from build123d import *

# Parameters (mm, degrees)
SKETCH_1_W      = 22.5
SKETCH_1_H      = 12.5
EXTRUDE_1_DEPTH = 17
SKETCH_2_W      = 32
SKETCH_2_H      = 12.5
SKETCH_2_R      = 1.5
EXTRUDE_2_DEPTH = 1.5
SKETCH_3_W      = 22.5
SKETCH_3_H      = 12.5
EXTRUDE_3_DEPTH = 4
SKETCH_4_R      = 5.5
EXTRUDE_4_DEPTH = 6.5
SKETCH_5_R      = 2.5
EXTRUDE_5_DEPTH = 3.5


with BuildPart() as part:
    # 草图1 → 凸台-拉伸1 (new body)
    with BuildSketch(Plane(origin=(0, 0, 0), x_dir=(1, 0, 0), z_dir=(0, 1, 0))):
        with Locations((11.25, -6.25)):
            Rectangle(SKETCH_1_W, SKETCH_1_H)
    extrude(amount=EXTRUDE_1_DEPTH)

    # 草图2 → 凸台-拉伸2 (add)
    with BuildSketch(Plane(origin=(0, 17, 0), x_dir=(1, 0, 0), z_dir=(0, 1, 0))):
        with Locations((11.25, -6.25)):
            Rectangle(SKETCH_2_W, SKETCH_2_H)
        with Locations(Location((-2.75, -6.25, 0), (0, 0, 270))):
            Circle(SKETCH_2_R, mode=Mode.SUBTRACT)
        with Locations(Location((25.25, -6.25, 0), (0, 0, 270))):
            Circle(SKETCH_2_R, mode=Mode.SUBTRACT)
    extrude(amount=EXTRUDE_2_DEPTH)

    # 草图3 → 凸台-拉伸3 (add)
    with BuildSketch(Plane(origin=(0, 18.5, 0), x_dir=(1, 0, 0), z_dir=(0, 1, 0))):
        with Locations((11.25, -6.25)):
            Rectangle(SKETCH_3_W, SKETCH_3_H)
    extrude(amount=EXTRUDE_3_DEPTH)

    # 草图4 → 凸台-拉伸4 (add)
    with BuildSketch(Plane(origin=(0, 22.5, 0), x_dir=(1, 0, 0), z_dir=(0, 1, 0))):
        with Locations(Location((17.25, -6.25, 0), (0, 0, 17.341442803))):
            Circle(SKETCH_4_R)
    extrude(amount=EXTRUDE_4_DEPTH)

    # 草图5 → 凸台-拉伸5 (add)
    with BuildSketch(Plane(origin=(0, 29, 0), x_dir=(1, 0, 0), z_dir=(0, 1, 0))):
        with Locations(Location((17.25, -6.25, 0), (0, 0, 270))):
            Circle(SKETCH_5_R)
    extrude(amount=EXTRUDE_5_DEPTH)


solid = part.part
Could you check a few things on this model? Use its own coordinates, in mm. A direction names the side the tool comes from. Round coordinates to 2 decimals unless told otherwise and drop trailing zeros. Loops run counter-clockwise (first coordinate to the right, second up) from the corner with the lowest first, then second, coordinate; pieces in that order, holes last. Notation, with made-up numbers: (-35, 18.5) - (-6, 18.5) arc R12 cw to (-6, 25.5) - close; hole circle Ø9 at (85.5, 39.25). An arc over 180 degrees is marked (long way). Write item = value, one per line.
1) I need wall thicknesses on line 1 along X through (y, z) = (17.9, 6.25); line 2 along Y through (x, z) = (-1.5, 2.75); line 3 along Y through (x, z) = (19.5, 11.5). Which ranges of each line are inside material? Lowest first, please. Write a range as from..to.
Computed:
line_1 = -4.75..-4.25, -1.25..23.75, 26.75..27.25
line_2 = 17..18.5
line_3 = 0..22.5
2) Imagine slicing it at B-B (x = -2.75). Please give me the cut outline in (y, z).
Computed:
outline = (17, 0) - (18.5, 0) - (18.5, 4.75) - (17, 4.75) - close; (17, 7.75) - (18.5, 7.75) - (18.5, 12.5) - (17, 12.5) - close
3) Imagine slicing it at C-C (y = 28.5). Please give me the cut outline in (x, z), and give its area (3 significant figures).
Computed:
outline = circle Ø11 at (17.25, 6.25)
area = 95.0 mm2
4) Imagine slicing it at D-D (x = 17.25). Please give me the cut outline in (y, z), and give its area (3 significant figures).
Computed:
outline = (0, 0) - (22.5, 0) - (22.5, 0.75) - (29, 0.75) - (29, 3.75) - (32.5, 3.75) - (32.5, 8.75) - (29, 8.75) - (29, 11.75) - (22.5, 11.75) - (22.5, 12.5) - (0, 12.5) - close
area = 370 mm2
5) On a 3-axis mill with a long thin cutter (end or side, diameter ignored), from which of +Z, -Z, +X, -X, +Y, -Y can I reach the whole of each face in a straight line? I mean faces 1 (the flat face through (0, 20, 6)), 2 (the flat face through (22.5, 20, 6)), 3 (the cylindrical face through (19.36, 30.73, 7.59)). Say none if no direction works.
Computed:
face_1 = +Z, -Z, -X, +Y
face_2 = +Z, -Z, +X
face_3 = +Y
6) If we mould it in two halves opening along Z, with no side actions, what happens to faces 4 (the flat face through (-1.9, 17, 4.8)), 5 (the flat face through (11, 11, 0)), 6 (the cylindrical face through (26.737, 17.74, 6.055)), 7 (the cylindrical face through (11.933, 25.704, 7.657))? For each: pulls with the +Z half, pulls with the -Z half, needs draft (parallel to the pull), parting line crosses it, or undercut.
Computed:
face_4 = needs draft
face_5 = pulls with the -Z half
face_6 = undercut
face_7 = parting line crosses it
7) I'm going to push flat-ended pins straight in: P1, Ø1.4, axis at x = 24.5, z = 3.5, coming from the +Y side; P2, Ø2, axis at y = 20, z = 6, coming from the -X side; P3, Ø6, axis at y = 11.5, z = 4.5, coming from the +X side. Where does each tip first touch, or does it pass through?
Computed:
P1 = 18.5
P2 = 0
P3 = 22.5
8) Imagine slicing it at A-A (z = 6.25). Please give me the cut outline in (x, y), and give its area (4 significant figures).
Computed:
outline = (-4.75, 17) - (-4.25, 17) - (-4.25, 18.5) - (-4.75, 18.5) - close; (-1.25, 17) - (0, 17) - (0, 0) - (22.5, 0) - (22.5, 17) - (23.75, 17) - (23.75, 18.5) - (22.5, 18.5) - (22.5, 22.5) - (22.75, 22.5) - (22.75, 29) - (19.75, 29) - (19.75, 32.5) - (14.75, 32.5) - (14.75, 29) - (11.75, 29) - (11.75, 22.5) - (0, 22.5) - (0, 18.5) - (-1.25, 18.5) - close; (26.75, 17) - (27.25, 17) - (27.25, 18.5) - (26.75, 18.5) - close
area = 600.5 mm2
